from build123d import *

# Parameters (mm, degrees)
F0_R     = 10
F1_DEPTH = 25
F2_DEPTH = 50
F3_SIZE  = 2
F4_R     = 53.910386
F6_DEPTH = 50


with BuildPart() as f1:
    # F0 (on Front) → F1 (new body)
    with BuildSketch(Plane.XZ):
        with BuildLine():
            ThreePointArc((2.083333, -24.913043), (18.399502, -16.92508), (25, 0))
            ThreePointArc((25, 0), (18.399502, 16.92508), (2.083333, 24.913043))
            ThreePointArc((2.083333, 24.913043), (-25, 0), (2.083333, -24.913043))
        make_face()
        Circle(F0_R, mode=Mode.SUBTRACT)
        with BuildLine():
            ThreePointArc((2.083333, 24.913043), (18.399502, 16.92508), (25, 0))
            ThreePointArc((25, 0), (18.399502, -16.92508), (2.083333, -24.913043))
            Line((2.083333, -24.913043), (91.458333, -17.43913))
            ThreePointArc((91.458333, -17.43913), (72.5, 0), (91.458333, 17.43913))
            Line((91.458333, 17.43913), (2.083333, 24.913043))
        make_face()
        with BuildLine():
            ThreePointArc((107.5, 0), (102.879651, 11.847556), (91.458333, 17.43913))
            ThreePointArc((91.458333, 17.43913), (72.5, 0), (91.458333, -17.43913))
            ThreePointArc((91.458333, -17.43913), (102.879651, -11.847556), (107.5, 0))
        make_face()
        with Locations((90, 0)):
            Circle(F0_R, mode=Mode.SUBTRACT)
    extrude(amount=F1_DEPTH)

    # F0 (on Front) → F2 (join)
    with BuildSketch(Plane.XZ):
        with BuildLine():
            ThreePointArc((2.083333, -24.913043), (18.399502, -16.92508), (25, 0))
            ThreePointArc((25, 0), (18.399502, 16.92508), (2.083333, 24.913043))
            ThreePointArc((2.083333, 24.913043), (-25, 0), (2.083333, -24.913043))
        make_face()
        Circle(F0_R, mode=Mode.SUBTRACT)
    extrude(amount=F2_DEPTH)

    # F3
    f3_edges = [f1.edges().sort_by_distance(p)[0] for p in [
        (-2.083333, -50, 24.913043),
        (-10, -50, 0),
        (80, -25, 0),
    ]]
    chamfer(f3_edges, length=F3_SIZE)

    # F4 (on Front) → F6 (join)
    with BuildSketch(Plane.XZ):
        with Locations((-48.911478, 44.221319)):
            Circle(F4_R)
    extrude(amount=F6_DEPTH)


solid = f1.part
Read the model definition and answer for the solid it produces. Units are mm, in the model's axes. Give positions to 0.01 mm unless a question says otherwise; leave off trailing zeros. Loops run counter-clockwise (first coordinate to the right, second up) from the corner with the lowest first, then second, coordinate; pieces in that order, holes last. Notation, with made-up numbers: (77.5, 80.5) -> (112.5, 80.5) arc R16 cw to (112.5, 85.5) -> close; hole circle Ø8 at (19, 51). An arc over 180 degrees is marked (long way). Use a Markdown table: item, result.
Q1. Section C-C, the plane x = 36 is taken. Determine the outline of the cut face in (y, z).
Solved:
| item | result |
|---|---|
| outline | (-25, -22.08) -> (0, -22.08) -> (0, 22.08) -> (-25, 22.08) -> close |
Q2. Section A-A, the plane y = -8 is taken. Determine the outline of the cut face in (x, z).
Solved:
| item | result |
|---|---|
| outline | (-24.69, -3.94) arc R25 ccw to (2.08, -24.91) -> (91.46, -17.44) arc R17.5 ccw to (91.46, 17.44) -> (2.08, 24.91) arc R25 ccw to (1.44, 24.96) arc R53.91 ccw (long way) to start; hole circle Ø20 at (0, 0); hole circle Ø20 at (90, 0) |
Q3. Section D-D, the plane z = -6 is taken. Count the separate pieces of the cut face and the enclosed holes in it, then the cut area to 3 significant figures.
Solved:
| item | result |
|---|---|
| separate pieces | 4 |
| enclosed holes | 0 |
| area | 5,230 mm^2 |
Q4. Determine the mould class of faces 1 (the face through (54, -25, 0)), 2 (the face through (80, -11, 0)), 3 (the face through (47.396, -12.325, 21.124)) for opening direction X: pulls with the +X half, pulls with the -X half, needs draft (parallel to the pull), parting line crosses it, or undercut.
Solved:
| item | result |
|---|---|
| face 1 | needs draft |
| face 2 | undercut |
| face 3 | pulls with the +X half |
Q5. Find the intervals of material crossed by line 1 along X through (y, z) = (-7.5, 3.5); line 2 along X through (y, z) = (-14.5, 0.5); line 3 along Y through (x, z) = (19, 23), in increasing order.
Solved:
| item | result |
|---|---|
| line 1 | x = -84.24 to -9.37, 9.37 to 80.63, 99.37 to 107.15 |
| line 2 | x = -80.45 to -9.99, 9.99 to 80.01, 99.99 to 107.49 |
| line 3 | y = -25 to 0 |
Q6. Section B-B, the plane y = -30.5 is taken. Determine the outline of the cut face in (x, z), then the cut area to 3 significant figures.
Solved:
| item | result |
|---|---|
| outline | (-24.69, -3.94) arc R25 ccw to (2.08, -24.91) arc R25 ccw to (25, 0) arc R25 ccw to (2.08, 24.91) arc R25 ccw to (1.44, 24.96) arc R53.91 ccw (long way) to start; hole circle Ø20 at (0, 0) |
| area | 10,400 mm^2 |
Q7. Each of these flat-tipped pins is pushed along its axis until it touches: pin 1 (10 mm diameter, centred on y = -18.5, z = 83.5, fed in from -X); pin 2 (1.5 mm diameter, centred on y = -30.5, z = 12, fed in from +X); pin 3 (5 mm diameter, centred on y = -10, z = 39.5, fed in from +X); pin 4 (18 mm diameter, centred on x = 0, z = 0, fed in from -Y). Where does it stop, or does it pass through?
Solved:
| item | result |
|---|---|
| pin 1 | stops at x = -90.52 |
| pin 2 | stops at x = 22.33 |
| pin 3 | stops at x = 4.95 |
| pin 4 | passes through |
